from build123d import *

# Parameters (mm, degrees)
F0_W     = 35
F0_H     = 70
F0_R     = 3.95
F1_DEPTH = 30
F2_SIZE  = 4
F3_R     = 1
F4_DEPTH = 25


with BuildPart() as f1:
    # F0 (on Top) → F1 (new body)
    with BuildSketch(Plane.XY):
        Rectangle(F0_W, F0_H)
        with Locations((0, -15)):
            Circle(F0_R, mode=Mode.SUBTRACT)
        with Locations((0, 15)):
            Circle(F0_R, mode=Mode.SUBTRACT)
    extrude(amount=F1_DEPTH)

    # F2
    f2_edges = [f1.edges().sort_by_distance(p)[0] for p in [
        (0, 35, 30),
        (17.5, 0, 30),
        (-17.5, 0, 30),
        (17.5, 35, 15),
        (-17.5, 35, 15),
    ]]
    chamfer(f2_edges, length=F2_SIZE)

    # F3 (on face) → F4 (cut)
    with BuildSketch(Plane.XZ.offset(35)):
        with Locations((0, 15)):
            Circle(F3_R)
    extrude(amount=-F4_DEPTH, mode=Mode.SUBTRACT)


solid = f1.part
Could you check a few things on this model? Use its own coordinates, in mm. A direction names the side the tool comes from. Coordinates: 2 decimals unless noted, no trailing zeros. Order: outer loops, then holes, each group sorted by start corner. A loop starts at its lowest first (then second) coordinate and runs counter-clockwise, first axis right, second up. Notation, with made-up numbers: (42, 37) -> (63, 37) arc R12 cw to (63, 54) -> close; hole circle Ø8 at (41, 75). An arc over 180 degrees is marked (long way). One line per question, with ' | ' between items.
Q1. Imagine slicing it at D-D on y = -15. Please give me the cut outline in (x, z).
Return value:
outline: (-17.5, 0) -> (-3.95, 0) -> (-3.95, 30) -> (-13.5, 30) -> (-17.5, 26) -> close; (3.95, 0) -> (17.5, 0) -> (17.5, 26) -> (13.5, 30) -> (3.95, 30) -> close
Q2. I'm going to push a flat-ended pin straight in: P1, Ø6.5, axis at x = 0, y = -15, coming from the -Z side. Where does the tip first touch, or does it pass through?
Return value:
P1: through
Q3. Thinking about a two-plate mould opening in Z: for faces 1 (the face through (0, -2, 30)), 2 (the face through (0, -35, 11)), 3 (the face through (0, -10, 15)), 4 (the face through (0, 0, 0)), which applies, pulls with the +Z half, pulls with the -Z half, needs draft (parallel to the pull), parting line crosses it, or undercut?
Return value:
face 1: pulls with the +Z half | face 2: needs draft | face 3: undercut | face 4: pulls with the -Z half
Q4. Imagine slicing it at C-C on z = 15. Please give me the cut outline in (x, y), and give its area (3 significant figures).
Return value:
outline: (-17.5, -35) -> (-1, -35) -> (-1, -18.82) arc R3.95 cw to (-1, -11.18) -> (-1, -10) -> (1, -10) -> (1, -11.18) arc R3.95 cw to (1, -18.82) -> (1, -35) -> (17.5, -35) -> (17.5, 31) -> (13.5, 35) -> (-13.5, 35) -> (-17.5, 31) -> close; hole circle Ø7.9 at (0, 15) | area: 2,300 mm²
Q5. On a 3-axis mill with a long thin cutter (end or side, diameter ignored), from which of +Z, -Z, +X, -X, +Y, -Y can I reach the whole of each face in a straight line? I mean faces 5 (the face through (15, 32.2, 27.3)), 6 (the face through (0, -27, 14)). Say none if no direction works.
Return value:
face 5: +Z, +X, +Y | face 6: -Y
Q6. Imagine slicing it at B-B on z = 9.5. Please give me the cut outline in (x, y).
Return value:
outline: (-17.5, -35) -> (17.5, -35) -> (17.5, 31) -> (13.5, 35) -> (-13.5, 35) -> (-17.5, 31) -> close; hole circle Ø7.9 at (0, -15); hole circle Ø7.9 at (0, 15)
Q7. Imagine slicing it at A-A on x = 0. Please give me the cut outline in (y, z), and give its area (3 significant figures).
Return value:
outline: (-35, 0) -> (-18.95, 0) -> (-18.95, 14) -> (-35, 14) -> close; (-35, 16) -> (-18.95, 16) -> (-18.95, 30) -> (-35, 30) -> close; (-11.05, 0) -> (11.05, 0) -> (11.05, 30) -> (-11.05, 30) -> (-11.05, 16) -> (-10, 16) -> (-10, 14) -> (-11.05, 14) -> close; (18.95, 0) -> (35, 0) -> (35, 26) -> (31, 30) -> (18.95, 30) -> close | area: 1,580 mm²
Q8. If I drill on L1, parallel to Y at x = 0, z = 11; L2, parallel to Z at x = 0, y = -10.35; L3, parallel to X at y = -10.8, z = 15, over which ranges is the centre line in solid material (lowest first)?
Return value:
L1: -35 to -18.95, -11.05 to 11.05, 18.95 to 35 | L2: 0 to 14, 16 to 30 | L3: -17.5 to -1, 1 to 17.5
